Geometry: see drawing. Coordinates: mm, zero at the bounding-box minimum. Give positions to 0.01 mm unless a question says otherwise; leave off trailing zeros. Order: outer loops, then holes, each group sorted by start corner. A loop starts at its lowest first (then second) coordinate and runs counter-clockwise, first axis right, second up. Notation, with made-up numbers: M -16.75,-8 L -11.75,-8 A32 cw -11.75,25 Z; hole C 3.5,38.25 d10. An arc over 180 degrees is marked long. Use a Markdown table: item, result.
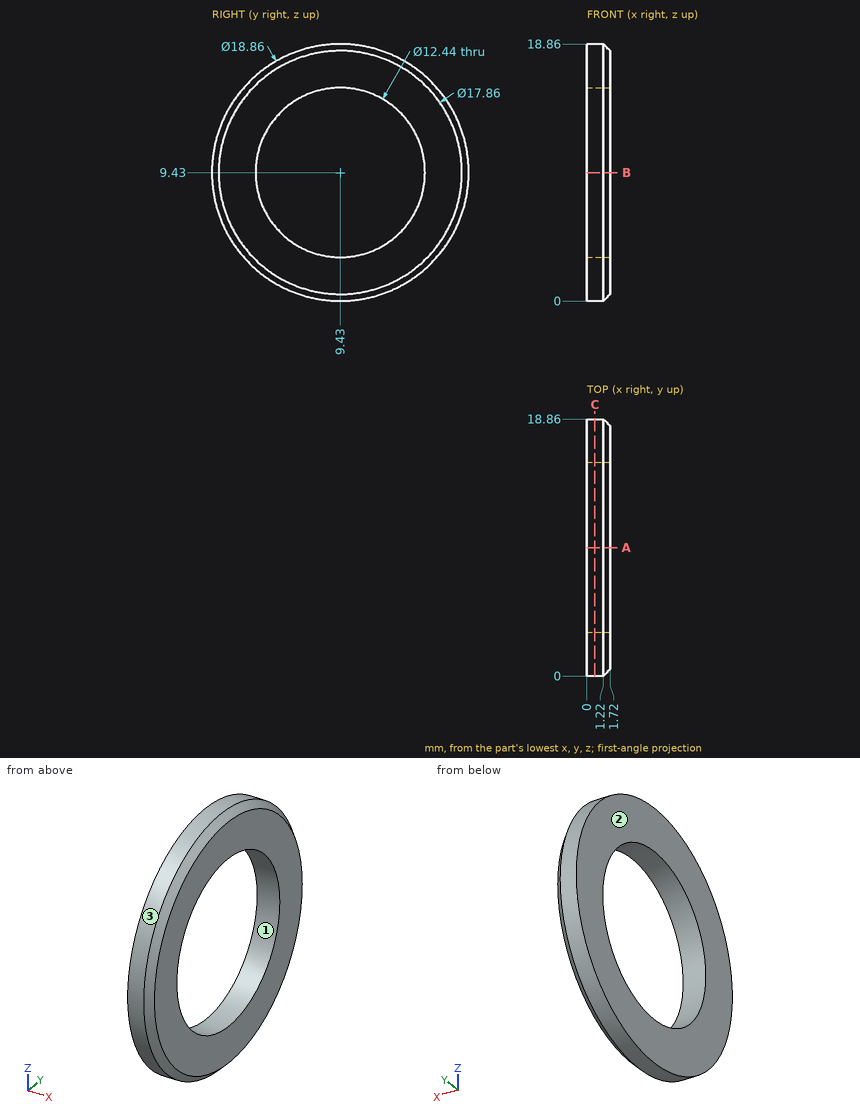
1) Mould query, pull axis Y, two halves, no side actions, for the marked faces 1, 2 and 3. Classes: released by +Y, released by -Y, zero draft, split by the parting line, or undercut.
Response values:
| item | result |
|---|---|
| face 1 | undercut |
| face 2 | zero draft |
| face 3 | split by the parting line |
2) Material intervals for line 1 (Z direction, x = 1.05, y = 9.43); line 2 (Z direction, x = 1.25, y = 9.43); line 3 (Y direction, x = 1.6, z = 12.25), sorted ascending. Write a range as from..to.
Response values:
| item | result |
|---|---|
| line 1 | z = 0..3.21, 15.65..18.86 |
| line 2 | z = 0.03..3.21, 15.65..18.83 |
| line 3 | y = 0.83..3.89, 14.97..18.03 |
3) First-contact query: pin 1 Ø1 at (x, y) = (0, 13.5) entering from +Z. Flat tip, straight axial feed; report the tip coordinate or a pass-through.
Response values:
| item | result |
|---|---|
| pin 1 | stops at z = 18.16 |
4) Cut plane A-A on y = 9.43. Return loops of the section in (x, z).
Response values:
| item | result |
|---|---|
| outline | M 0,0 L 1.22,0 L 1.72,0.5 L 1.72,3.21 L 0,3.21 Z; M 0,15.65 L 1.72,15.65 L 1.72,18.36 L 1.22,18.86 L 0,18.86 Z |
5) Cut plane C-C on x = 0.6. Return loops of the section in (y, z), and give its area (3 significant figures).
Response values:
| item | result |
|---|---|
| outline | C 9.43,9.43 d18.86; hole C 9.43,9.43 d12.44 |
| area | 158 mm² |
